```python
from build123d import *

# Parameters (mm, degrees)
SKETCH1_W           = 128
SKETCH1_H           = 278
BOSS_EXTRUDE1_DEPTH = 6.35
SKETCH2_W           = 16
SKETCH2_H           = 42
SKETCH2_H_2         = 45
SKETCH2_H_3         = 15
CUT_EXTRUDE1_DEPTH  = 31.7625
SKETCH5_R           = 1.6
CUT_EXTRUDE3_DEPTH  = 10


with BuildPart() as part:
    # Sketch1 → Boss-Extrude1 (new body)
    with BuildSketch(Plane.XY):
        with Locations((64, 139)):
            Rectangle(SKETCH1_W, SKETCH1_H)
    extrude(amount=BOSS_EXTRUDE1_DEPTH)

    # Sketch2 → Cut-Extrude1 (cut)
    with BuildSketch(Plane.XY.offset(6.35)):
        with Locations((8, 257)):
            Rectangle(SKETCH2_W, SKETCH2_H)
        with Locations((120, 255.5)):
            Rectangle(SKETCH2_W, SKETCH2_H_2)
        with Locations((120, 7.5)):
            Rectangle(SKETCH2_W, SKETCH2_H_3)
        with Locations((8, 7.5)):
            Rectangle(SKETCH2_W, SKETCH2_H_3)
    extrude(amount=-CUT_EXTRUDE1_DEPTH, mode=Mode.SUBTRACT)

    # Sketch5 → Cut-Extrude3 (cut)
    with BuildSketch(Plane.XY.offset(6.35)):
        with Locations((24, 257.75)):
            Circle(SKETCH5_R)
        with Locations((95, 257.75)):
            Circle(SKETCH5_R)
        with Locations((87.5, 210.5)):
            Circle(SKETCH5_R)
        with Locations((115.5, 210.5)):
            Circle(SKETCH5_R)
        with Locations((87.5, 141.5)):
            Circle(SKETCH5_R)
        with Locations((115.5, 141.5)):
            Circle(SKETCH5_R)
        with Locations((69.697400928, 118.75)):
            Circle(SKETCH5_R)
        with Locations((40.197400928, 228.25)):
            Circle(SKETCH5_R)
        with Locations((15, 211)):
            Circle(SKETCH5_R)
        with Locations((15, 166)):
            Circle(SKETCH5_R)
        with Locations((39, 8.308927031)):
            Circle(SKETCH5_R)
        with Locations((89, 8.308927031)):
            Circle(SKETCH5_R)
        with Locations((23, 100)):
            Circle(SKETCH5_R)
        with Locations((23, 42)):
            Circle(SKETCH5_R)
        with Locations((109, 42)):
            Circle(SKETCH5_R)
        with Locations((109, 100)):
            Circle(SKETCH5_R)
    extrude(amount=-CUT_EXTRUDE3_DEPTH, mode=Mode.SUBTRACT)


solid = part.part
```
Check sheet for the modelled part. Datum: model origin and axes. Units: mm. A direction names the side the tool comes from. Round coordinates to 2 decimals unless told otherwise and drop trailing zeros. Write each loop counter-clockwise with the first axis right and the second up, starting at its lowest first coordinate (ties: lowest second). Pieces come first, ordered by that corner, then holes. Notation, with made-up numbers: M -26,53.25 L -2,53.25 A31 cw -2,80.25 Z; hole C 76.25,-3 d1. An arc over 180 degrees is marked long. Write item = value, one per line. Start each with the question number.
1. Section check A-A, the plane z = 2.5. State how many separate pieces and enclosed holes the cut face has, then the cut area to 3 significant figures.
2. Scan lines: line 1 (Y direction, x = 15, z = 3.75); line 2 (Y direction, x = 108.5, z = 6); line 3 (Y direction, x = 95, z = 1.5). Record each from-to range of solid material in increasing order. Write a range as [from, to].
3. Gauge pin test, flat ends, axial feed: pin 1 (1.9 mm diameter, centred on y = 8, z = 4.5, fed in from -X); pin 2 (1.9 mm diameter, centred on x = 11.5, z = 2.5, fed in from -Y). Record the tip position at first contact, or that the pin passes through.
4. Tool access check on faces 1 (the flat face through (8, 236, 3)), 2 (the flat face through (63, 141, 6.35)), 3 (the flat face through (112, 255, 3)), 4 (the flat face through (16, 7, 3)), 5 (the flat face through (112, 7, 3)). Record the directions out of +Z, -Z, +X, -X, +Y, -Y that give a thin tool (end or side, any length) a straight path to the whole face; none if there is none.
5. Section check B-B, the plane y = 243. Record the cut outline in (x, z), then the cut area to 3 significant figures.
Results found:
q1.separate_pieces = 1
q1.enclosed_holes = 16
q1.area = 33,600 mm^2
q2.line_1 = [15, 164.4], [167.6, 209.4], [212.6, 236]
q2.line_2 = [0, 40.48], [43.52, 98.48], [101.52, 278]
q2.line_3 = [0, 256.15], [259.35, 278]
q3.pin_1 = 16
q3.pin_2 = 15
q4.face_1 = +Z, -Z, -X, +Y
q4.face_2 = +Z, +X, -X, +Y, -Y
q4.face_3 = +Z, -Z, +X, +Y
q4.face_4 = +Z, -Z, -X, -Y
q4.face_5 = +Z, -Z, +X, -Y
q5.outline = M 16,0 L 112,0 L 112,6.35 L 16,6.35 Z
q5.area = 610 mm^2
